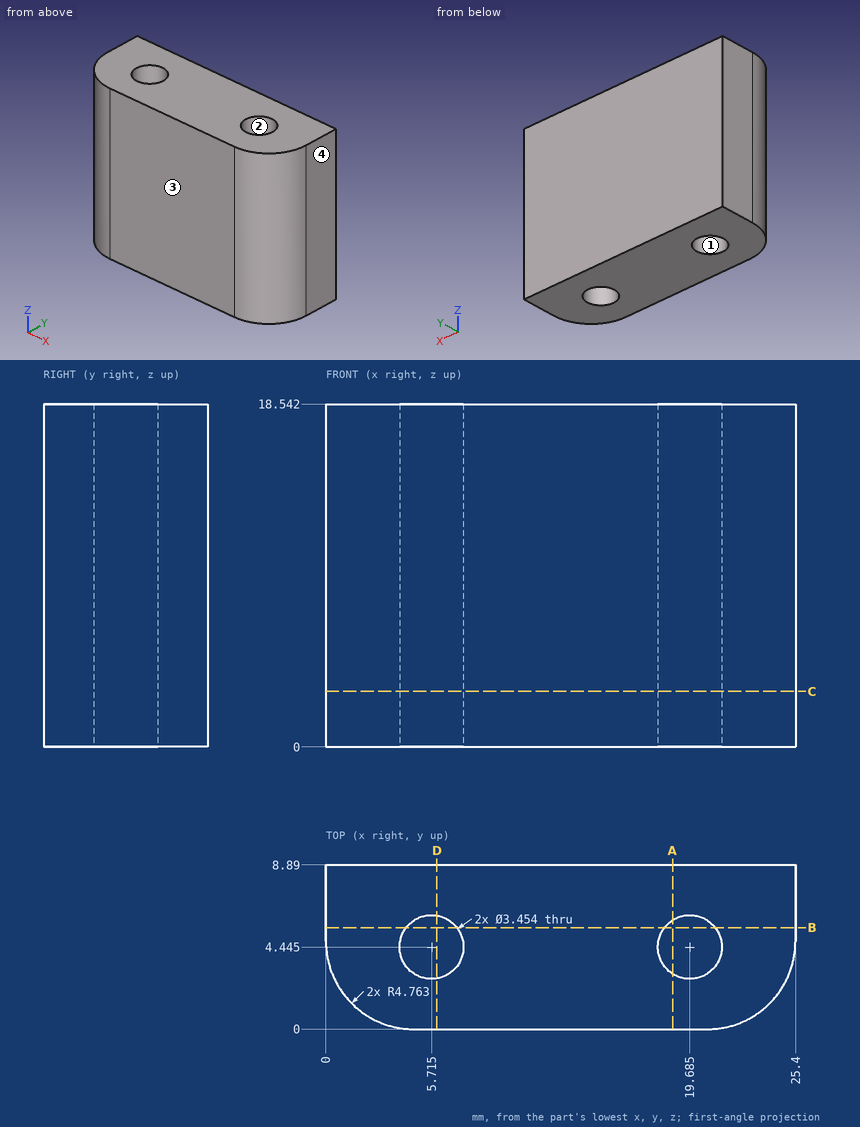
Job drawing, mm, ordinate dimensions from the low corner. One solid piece. Give positions to 0.01 mm unless a question says otherwise; leave off trailing zeros. Write each loop counter-clockwise with the first axis right and the second up, starting at its lowest first coordinate (ties: lowest second). Pieces come first, ordered by that corner, then holes. Notation, with made-up numbers: M 36.5,-28 L 64.5,-28 A13 ccw 64.5,-15 Z; hole C -36,80 d10. An arc over 180 degrees is marked long. One line per item, written item: value. Start each with the question number.
Q1. Saw through at C-C, the plane z = 3. Write the cut outline in (x, y) (1 decimal).
Q2. Probe probe 1 along X at (y, z) = (4.25, 13.5); probe 2 along X at (y, z) = (6, 13.75) (1 decimal); probe 3 along Y at (x, z) = (19.75, 7.5). List the from-to ranges inside material, lowest first. Write a range as [from, to].
Q3. Saw through at B-B, the plane y = 5.5. Write the cut outline in (x, z).
Q4. Two-plate mould, pull along Y, no slides. Class the marked faces 1, 2, 3 and 4: +Y half, -Y half, draft (parallel to the pull), parting line (faces both ways), or undercut.
Q5. Saw through at A-A, the plane x = 18.75. Write the cut outline in (y, z).
Q6. Drop a flat-ended pin along its axis: pin 1 Ø2 at (y, z) = (3, 13) entering from -X. Give the stop position or say it passes through.
Q7. Saw through at D-D, the plane x = 6. Write the cut outline in (y, z), plus the area to 3 significant figures.
Output values:
1. outline: M 0,4.8 A4.8 ccw 4.8,0 L 20.6,0 A4.8 ccw 25.4,4.8 L 25.4,8.9 L 0,8.9 Z; hole C 5.7,4.4 d3.5; hole C 19.7,4.4 d3.5
2. probe 1: x = [0.03, 4], [7.43, 17.97], [21.4, 25.37]
2. probe 2: x = [0, 5], [6.5, 18.9], [20.4, 25.4]
2. probe 3: y = [0, 2.72], [6.17, 8.89]
3. outline: M 0,0 L 4.35,0 L 4.35,18.54 L 0,18.54 Z; M 7.08,0 L 18.32,0 L 18.32,18.54 L 7.08,18.54 Z; M 21.05,0 L 25.4,0 L 25.4,18.54 L 21.05,18.54 Z
4. face 1: undercut
4. face 2: undercut
4. face 3: -Y half
4. face 4: draft
5. outline: M 0,0 L 2.99,0 L 2.99,18.54 L 0,18.54 Z; M 5.9,0 L 8.89,0 L 8.89,18.54 L 5.9,18.54 Z
6. pin 1: stops at x = 0.06
7. outline: M 0,0 L 2.74,0 L 2.74,18.54 L 0,18.54 Z; M 6.15,0 L 8.89,0 L 8.89,18.54 L 6.15,18.54 Z
7. area: 102 mm²
